```python
from build123d import *

# Parameters (mm, degrees)
SKETCH1_R                      = 1.7
BOSS_EXTRUDE1_DEPTH            = 8.74825
F_4_8_4_8_DIAMETER_HOLE1_D     = 4.8
F_4_8_4_8_DIAMETER_HOLE1_DEPTH = 6.4
F_4_8_4_8_DIAMETER_HOLE1_TIP   = 1.442065486
CHANFREIN3_SIZE                = 0.5
FILLET1_R                      = 3
CHANFREIN2_SIZE                = 2


with BuildPart() as part:
    # Sketch1 → Boss-Extrude1 (new body)
    with BuildSketch(Plane(origin=(0, 0, 0), x_dir=(1, 0, 0), z_dir=(0, 1, 0))):
        with BuildLine():
            ThreePointArc((-3.307377147, -6.731363636), (0, -16.4), (3.307377147, -6.731363636))
            ThreePointArc((3.307377147, -6.731363636), (6.143640332, -4.301823273), (7.456602343, -0.805655944))
            ThreePointArc((7.456602343, -0.805655944), (15.410958981, 5.609130351), (5.194223131, 5.410179855))
            ThreePointArc((5.194223131, 5.410179855), (0, 7.5), (-5.194223131, 5.410179855))
            ThreePointArc((-5.194223131, 5.410179855), (-15.410958981, 5.609130351), (-7.456602343, -0.805655944))
            ThreePointArc((-7.456602343, -0.805655944), (-6.143640332, -4.301823273), (-3.307377147, -6.731363636))
        make_face()
        with Locations(Location((0, -11, 0), (0, 0, 270))):
            Circle(SKETCH1_R, mode=Mode.SUBTRACT)
        with Locations(Location((-10.336618829, 3.762221577, 0), (0, 0, 270))):
            Circle(SKETCH1_R, mode=Mode.SUBTRACT)
        with Locations(Location((10.336618829, 3.762221577, 0), (0, 0, 270))):
            Circle(SKETCH1_R, mode=Mode.SUBTRACT)
    extrude(amount=-BOSS_EXTRUDE1_DEPTH)

    # Ø4.8 (4.8) Diameter Hole1
    with Locations(Plane(origin=(0, 0, 0), x_dir=(1, 0, 0), z_dir=(0, 1, 0))):
        with Locations((-10.336618829, 3.762221577), (10.336618829, 3.762221577), (0, -11)):
            Hole(F_4_8_4_8_DIAMETER_HOLE1_D / 2, depth=F_4_8_4_8_DIAMETER_HOLE1_DEPTH)
            with Locations((0, 0, -(F_4_8_4_8_DIAMETER_HOLE1_DEPTH + F_4_8_4_8_DIAMETER_HOLE1_TIP / 2))):  # 118° drill point
                Cone(0, F_4_8_4_8_DIAMETER_HOLE1_D / 2, F_4_8_4_8_DIAMETER_HOLE1_TIP, mode=Mode.SUBTRACT)

    # Chanfrein3
    chanfrein3_edges = [part.edges().sort_by_distance(p)[0] for p in [
        (2.4, 0, 11),
        (12.736618829, 0, -3.762221577),
        (-7.936618829, 0, -3.762221577),
    ]]
    chamfer(chanfrein3_edges, length=CHANFREIN3_SIZE)

    # Sketch2 → Cut-Revolve1 (revolve, cut)
    with BuildSketch(Plane(origin=(0, 0, 0), x_dir=(0, 0, -1), z_dir=(1, 0, 0)), mode=Mode.PRIVATE) as cut_revolve1_sk:
        Polygon((0, 0), (6, 0), (5.5, -0.5), (5.5, -4.5), (4.25, -4.5), (4.25, -6.5), (0, -6.5), align=None)
    revolve(cut_revolve1_sk.sketch.rotate(Axis((0, 1.69902052, 0), (0, -1, 0)), 180), axis=Axis((0, 1.69902052, 0), (0, -1, 0)), mode=Mode.SUBTRACT)

    # Fillet1
    fillet1_edges = [part.edges().sort_by_distance(p)[0] for p in [
        (3.307377147, -4.374125, 6.731363636),
        (-3.307377147, -4.374125, 6.731363636),
        (-7.456602343, -4.374125, 0.805655944),
        (-5.194223131, -4.374125, -5.410179855),
        (5.194223131, -4.374125, -5.410179855),
        (7.456602343, -4.374125, 0.805655944),
    ]]
    fillet(fillet1_edges, radius=FILLET1_R)

    # Chanfrein2
    chanfrein2_edges = [part.edges().sort_by_distance(p)[0] for p in [
        (0, -6.5, -4.25),
    ]]
    chamfer(chanfrein2_edges, length=CHANFREIN2_SIZE - 0.0001)  # a hair under: the kernel refuses the full size


solid = part.part
```
The model under review builds one solid part; all positions refer to its coordinate system, in mm. A direction names the side the tool comes from. Round coordinates to 2 decimals unless told otherwise and drop trailing zeros. Write each loop counter-clockwise with the first axis right and the second up, starting at its lowest first coordinate (ties: lowest second). Pieces come first, ordered by that corner, then holes.
(1) Wall thickness on L1, parallel to X at y = -3.25, z = -4.5; L2, parallel to Y at x = 0, z = 1.75; L3, parallel to X at y = -3.75, z = 3.5: over which ranges is each line inside the solid? List them lowest first.
(2) Mouldability with a two-part tool opening along Z and no side actions: class faces 1 (the cylindrical face through (-6.15, -4.31, 4.29)), 2 (the flat face through (0, -8.748, 1)), 3 (the cylindrical face through (-0.153, -4.313, 16.398)) as +Z half, -Z half, draft (parallel to the pull), parting line (faces both ways), or undercut.
(3) Machinability: for faces 4 (the cylindrical face through (15.461, -4.313, -5.464)), 5 (the cylindrical face through (-12.554, -3.491, -2.843)), which of the approach directions +Z, -Z, +X, -X, +Y, -Y give a long, thin tool a straight path to every point of the face, cutting with its end or side? Answer none if there is none.
(4) We need section D-D on y = -5.5. Give the number of separate pieces and of enclosed holes in the cut face, and give its area (3 significant figures).
(5) We need section B-B on z = 11. Give the boundary of the cut face in (x, y), and give its area (3 significant figures).
(6) Insertion check: pin 1 (3 mm diameter, centred on x = 10.34, z = -3.76, fed in from -Y); pin 2 (2.5 mm diameter, centred on x = 0.5, z = 1, fed in from +Y); pin 3 (5.5 mm diameter, centred on x = 0, z = 11, fed in from +Y); pin 4 (1 mm diameter, centred on y = -4, z = 0.5, fed in from +X). Each pin has a flat end and moves straight along its axis. Give the tip position at first contact, or say it passes through.
Findings below:
1. L1: x = -15.69 to -12.62, -8.05 to -3.16, 3.16 to 8.05, 12.62 to 15.69
1. L2: y = -8.75 to -6.5
1. L3: x = -6.63 to -4.24, 4.24 to 6.63
2. face 1: +Z half
2. face 2: draft
2. face 3: undercut
3. face 4: +Y, -Y
3. face 5: +Y
4. separate pieces: 1
4. enclosed holes: 4
4. area: 347 mm2
5. outline: (-5.4, -8.75) - (-1.7, -8.75) - (-1.7, -6.82) - (-2.4, -6.4) - (-2.4, -0.5) - (-2.9, 0) - (-5.4, 0) - close; (1.7, -8.75) - (5.4, -8.75) - (5.4, 0) - (2.9, 0) - (2.4, -0.5) - (2.4, -6.4) - (1.7, -6.82) - close
5. area: 55.2 mm2
6. pin 1: passes through
6. pin 2: stops at y = -6.38
6. pin 3: stops at y = -0.15
6. pin 4: stops at x = 14.21
